Check sheet for the drawn part. Datum: minimum x, y, z corner. Units: mm. A direction names the side the tool comes from. Coordinates: 2 decimals unless noted, no trailing zeros. Loops run counter-clockwise (first coordinate to the right, second up) from the corner with the lowest first, then second, coordinate; pieces in that order, holes last. Notation, with made-up numbers: (48.25, -27) - (68.25, -27) arc R31 cw to (68.25, 0) - close; hole circle Ø7 at (68.5, 7.5). An arc over 180 degrees is marked (long way). Write item = value, one per line. Start each with the question number.
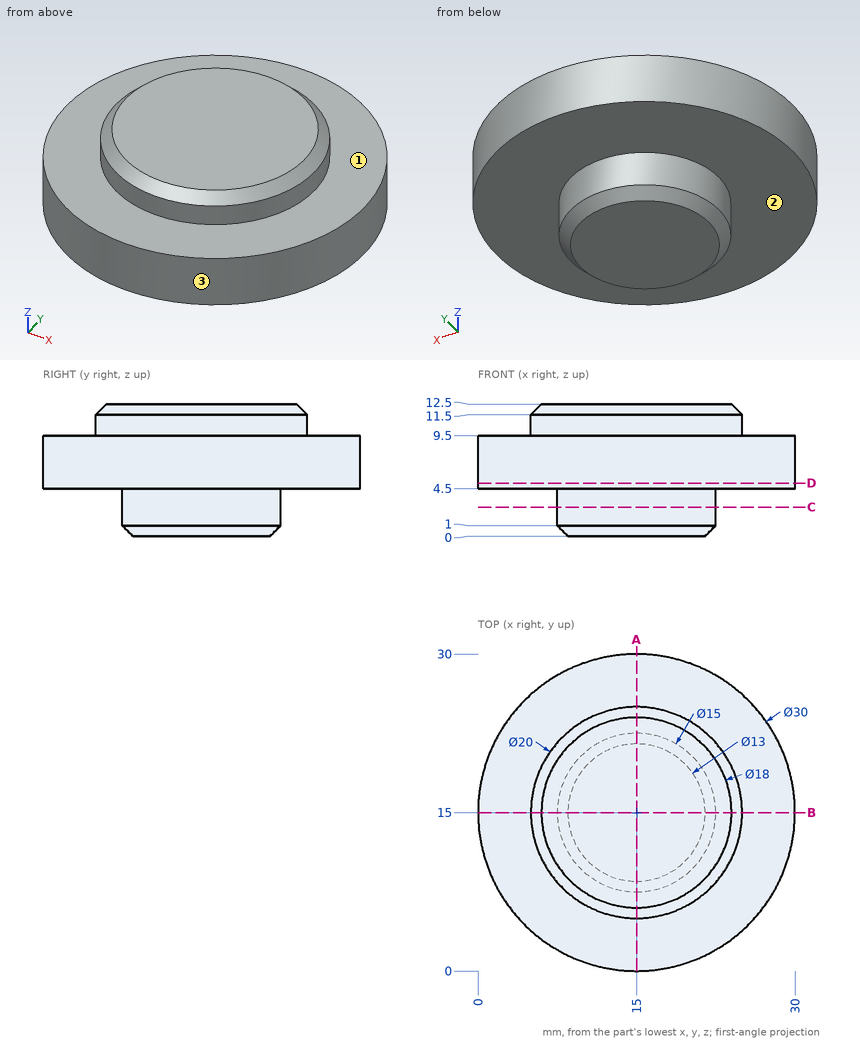
(1) Sectioned sample at D-D on z = 5. Enter the section's corners in (x, y), plus the area to 3 significant figures.
(2) Depth check by flat-ended pin: pin 1 (1 mm diameter, centred on x = 6, y = 13, fed in from -Z); pin 2 (3 mm diameter, centred on y = 4, z = 5, fed in from -X); pin 3 (4 mm diameter, centred on y = 23.5, z = 9, fed in from -X). Enter the tip coordinate at first touch or a pass-through.
(3) Sectioned sample at A-A on x = 15. Enter the section's corners in (y, z).
(4) Sectioned sample at C-C on z = 2.75. Enter the section's corners in (x, y), plus the area to 3 significant figures.
(5) Scan lines: line 1 (Z direction, x = 24.75, y = 23.25); line 2 (Z direction, x = 9.25, y = 21); line 3 (Y direction, x = 18.5, z = 10.5). Record each from-to range of solid material in increasing order.
(6) Tool access check on the marked faces 1, 2 and 3. Record the directions out of +Z, -Z, +X, -X, +Y, -Y that give a thin tool (end or side, any length) a straight path to the whole face; none if there is none.
Working result:
q1.outline = circle Ø30 at (15, 15)
q1.area = 707 mm2
q2.pin_1 = 4.5
q2.pin_2 = 3.39
q2.pin_3 = 1.48
q3.outline = (0, 4.5) - (7.5, 4.5) - (7.5, 1) - (8.5, 0) - (21.5, 0) - (22.5, 1) - (22.5, 4.5) - (30, 4.5) - (30, 9.5) - (25, 9.5) - (25, 11.5) - (24, 12.5) - (6, 12.5) - (5, 11.5) - (5, 9.5) - (0, 9.5) - close
q4.outline = circle Ø15 at (15, 15)
q4.area = 177 mm2
q5.line_1 = 4.5 to 9.5
q5.line_2 = 4.5 to 12.5
q5.line_3 = 5.63 to 24.37
q6.face_1 = +Z
q6.face_2 = -Z
q6.face_3 = +Z, -Z
